from build123d import *

# Parameters (mm, degrees)
PAD_DEPTH    = 10
SKETCH002_R  = 25
POCKET_DEPTH = 10.001


with BuildPart() as part:
    # Sketch → Pad (new body)
    with BuildSketch(Plane.XY):
        Polygon((0, 413.879036), (0, 452), (370, 452), (370, 0), (0, 0), align=None)
    extrude(amount=-PAD_DEPTH)

    # Sketch002 (on Face6 of Pad) → Pocket (cut, through all)
    with BuildSketch(Plane.XY):
        with Locations((300, 50)):
            Circle(SKETCH002_R)
    extrude(amount=-POCKET_DEPTH, mode=Mode.SUBTRACT)


solid = part.part
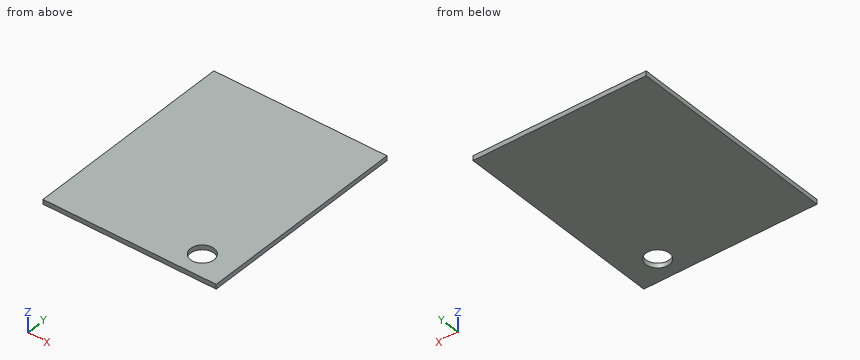
Read the model definition and answer for the solid it produces. Units are mm, in the model's axes. Round coordinates to 2 decimals unless told otherwise and drop trailing zeros. Loops run counter-clockwise (first coordinate to the right, second up) from the corner with the lowest first, then second, coordinate; pieces in that order, holes last.
Q1. Section B-B on x = 300 is taken. Write down the section's boundary in (y, z), and give its area (3 significant figures).
Q2. Section A-A on y = 50 is taken. Write down the section's boundary in (x, z), and give its area (3 significant figures).
Q3. Consider probe 1 along Y at (x, z) = (300, -3.5); probe 2 along X at (y, z) = (71, -2.5); probe 3 along Y at (x, z) = (277, -5). Determine where each line is inside the solid, lowest interval first.
Output:
1. outline: (0, -10) - (25, -10) - (25, 0) - (0, 0) - close; (75, -10) - (452, -10) - (452, 0) - (75, 0) - close
1. area: 4,020 mm2
2. outline: (0, -10) - (275, -10) - (275, 0) - (0, 0) - close; (325, -10) - (370, -10) - (370, 0) - (325, 0) - close
2. area: 3,200 mm2
3. probe 1: y = 0 to 25, 75 to 452
3. probe 2: x = 0 to 286.44, 313.56 to 370
3. probe 3: y = 0 to 40.2, 59.8 to 452
